from build123d import *

# Parameters (mm, degrees)
SKETCH1_R               = 70
BOSS_EXTRUDE1_DEPTH     = 5
SKETCH4_R               = 3
CUT_EXTRUDE2_DEPTH      = 100.121138008
CIRPATTERN1_COUNT       = 6
M6_CLEARANCE_HOLE1_D    = 6.6
SKETCH7_W               = 14
SKETCH7_H               = 5
CUT_EXTRUDE3_DEPTH      = 100.121138008
SKETCH8_R               = 1
SKETCH8_R_2             = 3.1
CUT_EXTRUDE4_DEPTH      = 100.121138008
F_1_2_CLEARANCE_HOLE1_D = 13.49248
FILLET1_R               = 0.5
SKETCH20_R              = 1.5
CUT_EXTRUDE6_DEPTH      = 100.121138008


with BuildPart() as part:
    # Sketch1 → Boss-Extrude1 (new body)
    with BuildSketch(Plane.XY):
        Circle(SKETCH1_R)
    extrude(amount=BOSS_EXTRUDE1_DEPTH)

    # Sketch4 → Cut-Extrude2 (cut, through all)
    with BuildSketch(Plane.XY):
        with Locations((0, 50)):
            Circle(SKETCH4_R)
    cut_extrude2 = extrude(amount=CUT_EXTRUDE2_DEPTH, mode=Mode.SUBTRACT)

    # CirPattern1: Cut-Extrude2 ×6 about axis
    cirpattern1_axis = Axis((0, 0, 0), (0, 0, 1))
    for i in range(1, CIRPATTERN1_COUNT):
        add(cut_extrude2.rotate(cirpattern1_axis, i * 360 / CIRPATTERN1_COUNT), mode=Mode.SUBTRACT)

    # M6 Clearance Hole1 (through all)
    with Locations(Plane.XY.offset(5)):
        with Locations((0, 50), (43.301270189, 25), (43.301270189, -25), (0, -50), (-43.301270189, -25), (-43.301270189, 25)):
            Hole(M6_CLEARANCE_HOLE1_D / 2)

    # Sketch7 → Cut-Extrude3 (cut, through all)
    with BuildSketch(Plane.XY):
        with Locations((2.5, -19.5)):
            Rectangle(SKETCH7_W, SKETCH7_H)
    extrude(amount=CUT_EXTRUDE3_DEPTH, mode=Mode.SUBTRACT)

    # Sketch8 → Cut-Extrude4 (cut, through all)
    with BuildSketch(Plane(origin=(0, 0, 0), x_dir=(-1, 0, 0), z_dir=(0, 0, -1))):
        with Locations((-2.5, 4)):
            Circle(SKETCH8_R)
        with Locations((-2.5, -17)):
            Circle(SKETCH8_R_2)
    extrude(amount=-CUT_EXTRUDE4_DEPTH, mode=Mode.SUBTRACT)

    # 1/2 Clearance Hole1 (through all)
    with Locations(Plane(origin=(0, 0, 0), x_dir=(-1, 0, 0), z_dir=(0, 0, -1))):
        with Locations((-2.5, 4)):
            Hole(F_1_2_CLEARANCE_HOLE1_D / 2)

    # Fillet1
    fillet1_edges = [part.edges().sort_by_distance(p)[0] for p in [
        (5.6, -17, 2.5),
        (-0.6, -17, 2.5),
    ]]
    fillet(fillet1_edges, radius=FILLET1_R)

    # Sketch20 → Cut-Extrude6 (cut, through all)
    with BuildSketch(Plane(origin=(0, 0, 0), x_dir=(-1, 0, 0), z_dir=(0, 0, -1))):
        with Locations((-8.5, -37)):
            Circle(SKETCH20_R)
        with Locations((3.5, -37)):
            Circle(SKETCH20_R)
    extrude(amount=-CUT_EXTRUDE6_DEPTH, mode=Mode.SUBTRACT)


solid = part.part
Verification items for the finished model (mm, model axes). A direction names the side the tool comes from. Coordinates: 2 decimals unless noted, no trailing zeros. Order: outer loops, then holes, each group sorted by start corner. A loop starts at its lowest first (then second) coordinate and runs counter-clockwise, first axis right, second up. Notation, with made-up numbers: M 61.25,-6 L 67.25,-6 A33 cw 67.25,33 Z; hole C 5,62.25 d8. An arc over 180 degrees is marked long. One line per item, written item: value. Start each with the question number.
Item 1: Sectioned sample at C-C on y = 25. Record the cut outline in (x, z).
Item 2: Sectioned sample at B-B on z = 0.85. Give the number of separate pieces and of enclosed holes in the cut face, then the cut area to 3 significant figures.
Item 3: Depth check by flat-ended pin: P1, Ø2.5, axis at x = -3.5, z = 3, coming from the -Y side; P2, Ø3, axis at y = 17.5, z = 3, coming from the +X side; P3, Ø2.5, axis at x = -3.5, y = -37, coming from the +Z side; P4, Ø1.7, axis at x = 7, z = 3, coming from the -Y side. Enter the tip coordinate at first touch or a pass-through.
Item 4: Access from +Z, -Z, +X, -X, +Y, -Y to the whole of each face (thin tool, end or side, straight path). Record for faces 4 (the flat face through (-1, -15, 0)), 5 (the flat face through (9.5, -20, 2)).
Item 5: Thickness scan on probe 1 along Y at (x, z) = (0, 2.35); probe 2 along Y at (x, z) = (-3.5, 2.95); probe 3 along X at (y, z) = (1.5, 4.55). Record the ranges inside material, lowest first.
Item 6: Sectioned sample at D-D on x = -60.5. Record the cut outline in (y, z).
Item 7: Mould release check, pull along X, two halves, no side actions. Record for faces 1 (the cylindrical face through (-55.55, -42.594, 2.465)), 2 (the flat face through (-1, -15, 5)), 3 (the flat face through (2, -22, 2)): pulls with the +X half, pulls with the -X half, needs draft (parallel to the pull), parting line crosses it, or undercut.
Item 8: Sectioned sample at A-A on y = 50. Record the cut outline in (x, z).
Calculated:
1. outline: M -65.38,0 L -46.6,0 L -46.6,5 L -65.38,5 Z; M -40,0 L 40,0 L 40,5 L -40,5 Z; M 46.6,0 L 65.38,0 L 65.38,5 L 46.6,5 Z
2. separate pieces: 1
2. enclosed holes: 10
2. area: 14,900 mm^2
3. P1: y = -69.96
3. P2: x = 68.15
3. P3: through
3. P4: y = -69.73
4. face 4: -Z, +X, -X, +Y, -Y
4. face 5: +Z, -Z
5. probe 1: -70 to -53.3, -46.7 to -22, -15.17 to -2.27, 10.27 to 46.7, 53.3 to 70
5. probe 2: -69.91 to -38.5, -35.5 to -22, -17 to 0.92, 7.08 to 69.91
5. probe 3: -69.98 to -3.77, 8.77 to 69.98
6. outline: M -35.21,0 L 35.21,0 L 35.21,5 L -35.21,5 Z
7. face 1: parting line crosses it
7. face 2: needs draft
7. face 3: undercut
8. outline: M -48.99,0 L -3.3,0 L -3.3,5 L -48.99,5 Z; M 3.3,0 L 48.99,0 L 48.99,5 L 3.3,5 Z
